Geometry check sheet. Reference: the model listing, model coordinates, mm. A direction names the side the tool comes from. Round coordinates to 2 decimals unless told otherwise and drop trailing zeros. Write each loop counter-clockwise with the first axis right and the second up, starting at its lowest first coordinate (ties: lowest second). Pieces come first, ordered by that corner, then holes. Notation, with made-up numbers: (26, -17) - (76, -17) arc R18 cw to (76, -6) - close; hole circle Ø8 at (-3.5, 5). An arc over 180 degrees is marked (long way). Return JSON: item names as keys, results as strings. Group by question number.
from build123d import *

# Parameters (mm, degrees)
F1_DEPTH = 50
F2_R     = 25
F3_R     = 24.99999
F4_R     = 15
F5_DEPTH = 10
F6_R     = 18
F7_DEPTH = 15
F8_R     = 12
F9_DEPTH = 25


# Not quite as in the source:
# - a fillet or chamfer is up to 0.001 mm smaller than in the source, because OpenCascade refuses the exact size


with BuildPart() as f1:
    # F0 (on Front) → F1 (new body)
    with BuildSketch(Plane.XZ):
        Polygon((0, 80), (0, 0), (88, 0), (88, 10), (38, 10), (38, 34), (30, 34), (30, 10), (10, 10), (10, 80), align=None)
    extrude(amount=F1_DEPTH)

    # F2
    f2_edges = [f1.edges().sort_by_distance(p)[0] for p in [
        (88, -50, 5),
    ]]
    fillet(f2_edges, radius=F2_R)

    # F3 (radius 25 in the source; OpenCascade refuses exactly that, so slightly less here)
    f3_edges = [f1.edges().sort_by_distance(p)[0] for p in [
        (88, 0, 5),
    ]]
    fillet(f3_edges, radius=F3_R)

    # F4 (on face) → F5 (cut, through all)
    with BuildSketch(Plane.XY.offset(10)):
        with Locations((63, -25)):
            Circle(F4_R)
    extrude(amount=-F5_DEPTH, mode=Mode.SUBTRACT)

    # F6 (on face) → F7 (join)
    with BuildSketch(Plane.YZ.offset(10)):
        with Locations((-25, 56)):
            Circle(F6_R)
    extrude(amount=F7_DEPTH)

    # F8 (on face) → F9 (cut, through all)
    with BuildSketch(Plane.YZ.offset(25)):
        with Locations((-25, 56)):
            Circle(F8_R)
    extrude(amount=-F9_DEPTH, mode=Mode.SUBTRACT)


solid = f1.part
1. Tool access check on faces 1 (the face through (25, -13, 52)), 2 (the face through (17.395, -15.323, 71.178)), 3 (the face through (30, -25, 22)), 4 (the face through (20, -25, 10)), 5 (the face through (8, 0, 25)). Record the directions out of +Z, -Z, +X, -X, +Y, -Y that give a thin tool (end or side, any length) a straight path to the whole face; none if there is none.
2. Section check A-A (z = 56). Enter the section's corners in (x, y).
3. Mould release check, pull along X, two halves, no side actions. Record for faces 6 (the face through (80.871, -42.482, 5.07)), 7 (the face through (10, -25, 37)), 8 (the face through (34, -25, 0)): pulls with the +X half, pulls with the -X half, needs draft (parallel to the pull), parting line crosses it, or undercut.
4. Section check C-C (x = 8). Enter the section's corners in (y, z).
5. Section check B-B (y = -22). Enter the section's corners in (x, z).
6. Depth check by flat-ended pin: pin 1 Ø15 at (x, y) = (65, -34) entering from +Z; pin 2 Ø4 at (x, y) = (34.5, -37) entering from +Z; pin 3 Ø12 at (y, z) = (-34.5, 18.5) entering from +X. Enter the tip coordinate at first touch or a pass-through.
7. Material ranges on line 1 along Z through (x, y) = (13, -25); line 2 along X through (y, z) = (-2, 59.5); line 3 along X through (y, z) = (-26.5, 10.5), recorded low to high.
8. Section check D-D (z = 18.5). Enter the section's corners in (x, y).
Result sheet:
{
 "1": {"face 1": "+Z, +X, +Y, -Y", "face 2": "+X", "face 3": "+Z, +Y, -Y", "face 4": "+Y, -Y", "face 5": "+Z, -Z, +X, -X, +Y"},
 "2": {"outline": "(0, -50) - (10, -50) - (10, -43) - (25, -43) - (25, -37) - (0, -37) - close; (0, -13) - (25, -13) - (25, -7) - (10, -7) - (10, 0) - (0, 0) - close"},
 "3": {"face 6": "pulls with the +X half", "face 7": "undercut", "face 8": "needs draft"},
 "4": {"outline": "(-50, 0) - (0, 0) - (0, 80) - (-50, 80) - close; hole circle Ø24 at (-25, 56)"},
 "5": {"outline": "(0, 0) - (48.3, 0) - (48.3, 10) - (38, 10) - (38, 34) - (30, 34) - (30, 10) - (10, 10) - (10, 38.25) - (25, 38.25) - (25, 44.38) - (0, 44.38) - close; (0, 67.62) - (25, 67.62) - (25, 73.75) - (10, 73.75) - (10, 80) - (0, 80) - close; (77.7, 0) - (87.82, 0) - (87.82, 10) - (77.7, 10) - close"},
 "6": {"pin 1": "stops at z = 10", "pin 2": "stops at z = 34", "pin 3": "stops at x = 38"},
 "7": {"line 1": "z = 0 to 10, 38 to 44, 68 to 74", "line 2": "x = 0 to 10", "line 3": "x = 0 to 10, 30 to 38"},
 "8": {"outline": "(0, -50) - (10, -50) - (10, 0) - (0, 0) - close; (30, -50) - (38, -50) - (38, 0) - (30, 0) - close"}
}
